```python
from build123d import *

# Parameters (mm, degrees)
BOSS_EXTRUDE1_DEPTH = 10
SKETCH2_R           = 2
CUT_EXTRUDE1_DEPTH  = 8
FILLET1_R           = 5


with BuildPart() as part:
    # Sketch1 → Boss-Extrude1 (new body)
    with BuildSketch(Plane.XY):
        with BuildLine():
            Line((0, 0), (-105, 0))
            ThreePointArc((-105, 0), (-117.249623327, 6.342822149), (-119.139622366, 20.007102889))
            Line((-119.139622366, 20.007102889), (-110.875178831, 43.345171481))
            ThreePointArc((-110.875178831, 43.345171481), (-101.737771304, 55.416038879), (-87.309141554, 60))
            Line((-87.309141554, 60), (87.309141554, 60))
            ThreePointArc((87.309141554, 60), (101.737771304, 55.416038879), (110.875178831, 43.345171481))
            Line((110.875178831, 43.345171481), (119.139622366, 20.007102889))
            ThreePointArc((119.139622366, 20.007102889), (117.249623327, 6.342822149), (105, 0))
            Line((105, 0), (0, 0))
        make_face()
    extrude(amount=BOSS_EXTRUDE1_DEPTH)

    # Sketch2 → Cut-Extrude1 (cut)
    with BuildSketch(Plane.XY.offset(10)):
        with Locations((-70, 22)):
            Circle(SKETCH2_R)
        with Locations((-70, 38)):
            Circle(SKETCH2_R)
        with Locations(Location((70, 22, 0), (0, 0, 180))):
            Circle(SKETCH2_R)
        with Locations(Location((70, 38, 0), (0, 0, 180))):
            Circle(SKETCH2_R)
    extrude(amount=-CUT_EXTRUDE1_DEPTH, mode=Mode.SUBTRACT)

    # Fillet1
    fillet1_edges = [part.edges().sort_by_distance(p)[0] for p in [
        (-117.249623327, 6.342822149, 0),
        (-115.007400599, 31.676137185, 0),
        (-101.737771304, 55.416038879, 0),
        (0, 60, 0),
        (101.737771304, 55.416038879, 0),
        (115.007400599, 31.676137185, 0),
        (117.249623327, 6.342822149, 0),
        (-117.249623327, 6.342822149, 10),
        (-115.007400599, 31.676137185, 10),
        (-101.737771304, 55.416038879, 10),
        (0, 60, 10),
        (101.737771304, 55.416038879, 10),
        (115.007400599, 31.676137185, 10),
        (117.249623327, 6.342822149, 10),
        (0, 0, 0),
        (0, 0, 10),
    ]]
    fillet(fillet1_edges, radius=FILLET1_R - 0.0001)  # a hair under: the kernel refuses the full size


solid = part.part
```
The listing builds one solid part. Answer for the finished solid, in the listing's coordinates (mm). A direction names the side the tool comes from. Coordinates: 2 decimals unless noted, no trailing zeros. Order: outer loops, then holes, each group sorted by start corner. A loop starts at its lowest first (then second) coordinate and runs counter-clockwise, first axis right, second up. Notation, with made-up numbers: M 20,28.25 L 36,28.25 A28 ccw 36,51.25 Z; hole C 22,9 d8. An arc over 180 degrees is marked long. Answer as a JSON object with one key per item and string values. Group by question number.
1. Section A-A on z = 7.5 is taken. Write down the section's boundary in (x, y).
2. Determine the mould class of faces 1 (the flat face through (70, 22, 2)), 2 (the flat face through (2, 30, 10)), 3 (the cylindrical face through (-113.606, 31.364, 1.504)) for opening direction X: released by +X, released by -X, zero draft, split by the parting line, or undercut.
3. Flat-ended cylindrical pins translate along their axes: P1, Ø2.5, axis at x = -70, y = 22, coming from the +Z side; P2, Ø3, axis at x = 23.5, z = 7.5, coming from the -Y side. Find the tip coordinate at first contact, or state that the pin passes through.
4. Straight lines are drawn through the part: line 1 (Y direction, x = 70, z = 4.75); line 2 (Y direction, x = -70, z = 8.5); line 3 (X direction, y = 16, z = 1.75). For each, find the intervals that lie inside material, in ascending order.
5. A tool of negligible diameter and unlimited length cuts with its end or side. For faces 4 (the cylindrical face through (68.092, 21.399, 6.056)), 5 (the cylindrical face through (-113.606, 31.364, 8.496)), from which of +Z, -Z, +X, -X, +Y, -Y can it reach the whole face along a straight path? Write none if from no direction.
Values follow:
{
 "1": {"outline": "M -118.51,19.78 A14.33 ccw -105,0.67 L 105,0.67 A14.33 ccw 118.51,19.78 L 110.24,43.12 A24.33 ccw 87.31,59.33 L -87.31,59.33 A24.33 ccw -110.24,43.12 Z; hole C -70,22 d4; hole C -70,38 d4; hole C 70,22 d4; hole C 70,38 d4"},
 "2": {"face 1": "undercut", "face 2": "zero draft", "face 3": "released by -X"},
 "3": {"P1": "z = 2", "P2": "y = 0.1"},
 "4": {"line 1": "0.01 to 20, 24 to 36, 40 to 59.99", "line 2": "1.43 to 20, 24 to 36, 40 to 58.57", "line 3": "-118.76 to 118.76"},
 "5": {"face 4": "+Z", "face 5": "+Z, -X, +Y"}
}
